Geometry: final body of the model. Coordinates: model frame, mm. A direction names the side the tool comes from. Give positions to 0.01 mm unless a question says otherwise; leave off trailing zeros. Loops run counter-clockwise (first coordinate to the right, second up) from the corner with the lowest first, then second, coordinate; pieces in that order, holes last.
1. Section A-A, the plane z = 39.5. Output: boundary loops of the cut face in (x, y).
2. First-contact query: P1, Ø1.5, axis at y = -33.5, z = 79.5, coming from the -X side; P2, Ø17, axis at x = -14.5, z = 30, coming from the -Y side; P3, Ø2, axis at x = -63.5, z = 67, coming from the -Y side. Flat tips, straight axial feed; report the tip coordinate or a pass-through.
3. Material intervals for line 1 along Y through (x, z) = (0, 75); line 2 along X through (y, z) = (-26.5, 17); line 3 along Z through (x, y) = (-16.5, 2.5), sorted ascending.
4. Access query for faces 4 (the face through (-68, 36, 63.181)), 5 (the face through (-59, 59.815, 35)), 6 (the face through (-8, 5, 7.686)), 7 (the face through (-11, 0, 35)). Directions: +Z, -Z, +X, -X, +Y, -Y. A direction counts if a zero-diameter tool reaches every point of the face in a straight line with its end or side. Return the directions, or none.
5. Section B-B, the plane z = 67. Output: boundary loops of the cut face in (x, y).
6. Draft query along Y for faces 1 (the face through (-75, 0, 35)), 2 (the face through (-13.559, -61.06, 105.404)), 3 (the face through (5.42, -37.334, 47.273)). Return one class per face: +Y half, -Y half, draft (parallel to the pull), parting line (faces both ways), or undercut.
from build123d import *

# Parameters (mm, degrees)
F0_R     = 72.0614296005
F1_DEPTH = 105.8891117573
F3_D     = 50
F4_SIZE  = 10
F5_W     = 59.8151311278
F5_H     = 55.4952472448
F6_DEPTH = 78.7402912974


with BuildPart() as f1:
    # F0 (on Top) → F1 (new body)
    with BuildSketch(Plane.XY):
        Circle(F0_R)
    extrude(amount=F1_DEPTH)

    # F3 (through all)
    with Locations(Plane.XY.offset(105.8891117573)):
        with Locations((0, -12.928519398)):
            Hole(F3_D / 2)

    # F4
    f4_edges = [f1.edges().sort_by_distance(p)[0] for p in [
        (-72.06143, 0, 105.889112),
        (-25, -12.928519, 105.889112),
    ]]
    chamfer(f4_edges, length=F4_SIZE)

    # F5 (on Right) → F6 (join)
    with BuildSketch(Plane.YZ):
        with Locations((29.9075655639, 35.4334488511)):
            Rectangle(F5_W, F5_H)
    extrude(amount=-F6_DEPTH)


solid = f1.part
Answers below:
1. outline: (-78.74, 0) - (-72.06, 0) arc R72.06 ccw (long way) to (-40.19, 59.82) - (-78.74, 59.82) - close; hole (-21.4, 0) arc R25 ccw (long way) to (0, 12.07) - (0, 0) - close
2. P1: stops at x = -64.19
2. P2: stops at y = -71.81
2. P3: stops at y = -35.87
3. line 1: y = -72.06 to -37.93, 12.07 to 72.06
3. line 2: x = -67.01 to -21, 21 to 67.01
3. line 3: z = 7.69 to 63.18
4. face 4: +Z, -X, +Y
4. face 5: +Z, -Z, -X, +Y
4. face 6: -Z
4. face 7: +Z, -Z
5. outline: circle Ø144.12 at (0, 0); hole circle Ø50 at (0, -12.93)
6. face 1: -Y half
6. face 2: parting line
6. face 3: undercut
